Can you work these out from the model? Positions are in its coordinate system, mm. Round coordinates to 2 decimals unless told otherwise and drop trailing zeros. Loops run counter-clockwise (first coordinate to the right, second up) from the corner with the lowest first, then second, coordinate; pieces in that order, holes last. Notation, with made-up numbers: (79, 70) - (138, 70) arc R27 ccw to (138, 107) - close; hole circle Ø1 at (59.25, 33.25). An arc over 180 degrees is marked (long way). Answer as CSV lines item,"result".
```python
from build123d import *

# Parameters (mm, degrees)
STRUCTURAL_MEMBER1_DEPTH = 762


with BuildPart() as part:
    # Sketch1 → Structural Member1 (new body)
    with BuildSketch(Plane.ZY):
        with BuildLine():
            Line((-25.4, -38.1), (25.4, -38.1))
            ThreePointArc((25.4, -38.1), (34.380256121, -34.380256121), (38.1, -25.4))
            Line((38.1, -25.4), (38.1, 25.4))
            ThreePointArc((38.1, 25.4), (34.380256121, 34.380256121), (25.4, 38.1))
            Line((25.4, 38.1), (-25.4, 38.1))
            ThreePointArc((-25.4, 38.1), (-34.380256121, 34.380256121), (-38.1, 25.4))
            Line((-38.1, 25.4), (-38.1, -25.4))
            ThreePointArc((-38.1, -25.4), (-34.380256121, -34.380256121), (-25.4, -38.1))
        make_face()
        with BuildLine():
            Line((-25.4, -31.75), (25.4, -31.75))
            ThreePointArc((25.4, -31.75), (29.890128061, -29.890128061), (31.75, -25.4))
            Line((31.75, -25.4), (31.75, 25.4))
            ThreePointArc((31.75, 25.4), (29.890128061, 29.890128061), (25.4, 31.75))
            Line((25.4, 31.75), (-25.4, 31.75))
            ThreePointArc((-25.4, 31.75), (-29.890128061, 29.890128061), (-31.75, 25.4))
            Line((-31.75, 25.4), (-31.75, -25.4))
            ThreePointArc((-31.75, -25.4), (-29.890128061, -29.890128061), (-25.4, -31.75))
        make_face(mode=Mode.SUBTRACT)
    extrude(amount=STRUCTURAL_MEMBER1_DEPTH)


solid = part.part
```
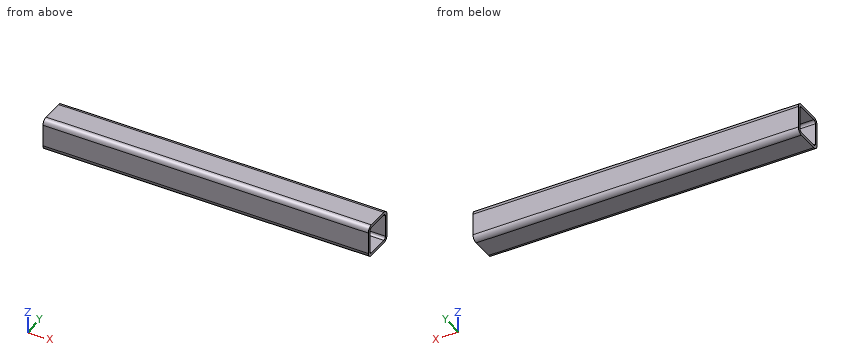
Q1. Imagine slicing it at A-A (x = -465). Write out the boundary of the cut face in (y, z), then the cut area to 3 significant figures.
Checks:
outline,"(-38.1, -25.4) arc R12.7 ccw to (-25.4, -38.1) - (25.4, -38.1) arc R12.7 ccw to (38.1, -25.4) - (38.1, 25.4) arc R12.7 ccw to (25.4, 38.1) - (-25.4, 38.1) arc R12.7 ccw to (-38.1, 25.4) - close; hole (-31.75, -25.4) arc R6.35 ccw to (-25.4, -31.75) - (25.4, -31.75) arc R6.35 ccw to (31.75, -25.4) - (31.75, 25.4) arc R6.35 ccw to (25.4, 31.75) - (-25.4, 31.75) arc R6.35 ccw to (-31.75, 25.4) - close"
area,"1,670 mm²"
Q2. I'm going to push flat-ended pins straight in: pin 1 Ø8 at (y, z) = (26, -26.5) entering from +X; pin 2 Ø1 at (x, y) = (-372.5, -30) entering from -Z. Where does each tip first touch, or does it pass through?
Checks:
pin 1,"through"
pin 2,"z = -37.42"
Q3. If I drill on line 1 along Y through (x, z) = (-584.5, -7.5); line 2 along Z through (x, y) = (-297, 27.5), over which ranges is the centre line in solid material (lowest first)? Write a range as [from, to].
Checks:
line 1,"[-38.1, -31.75], [31.75, 38.1]"
line 2,"[-37.93, -31.39], [31.39, 37.93]"
Q4. Imagine slicing it at B-B (y = -6.5). Write out the boundary of the cut face in (x, z), then the cut area to 3 significant figures.
Checks:
outline,"(-762, -38.1) - (0, -38.1) - (0, -31.75) - (-762, -31.75) - close; (-762, 31.75) - (0, 31.75) - (0, 38.1) - (-762, 38.1) - close"
area,"9,680 mm²"
